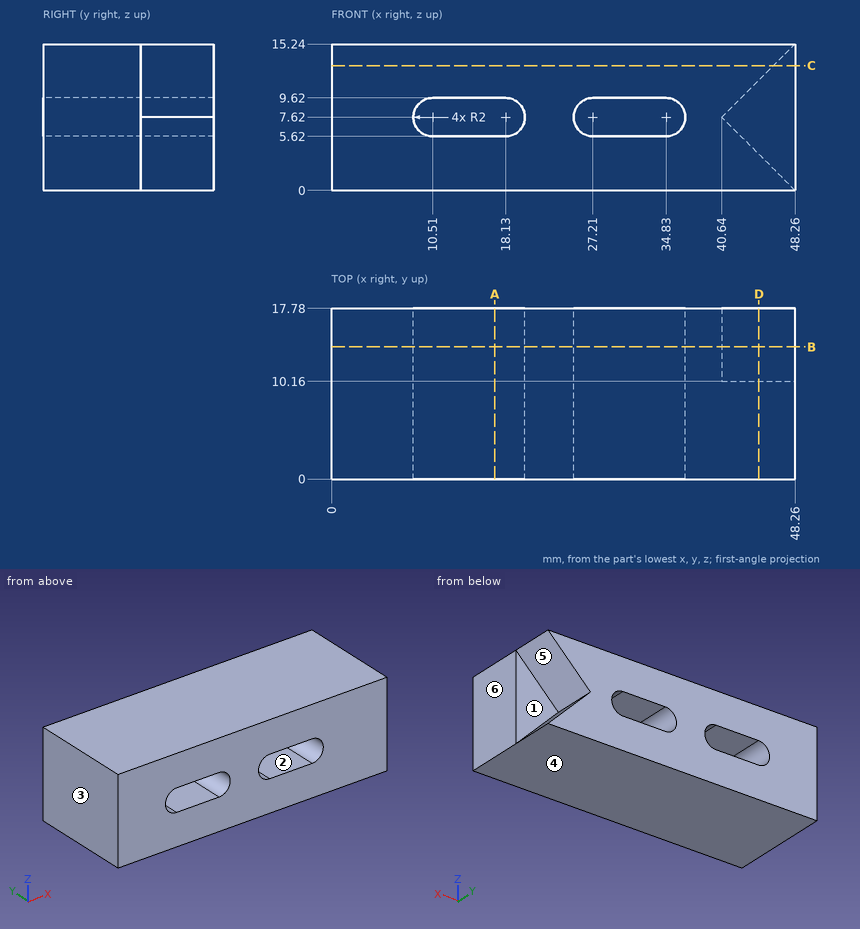
Part print with two shaded views. Sizes in mm from the minimum x, y, z corner. A direction names the side the tool comes from. Round coordinates to 2 decimals unless told otherwise and drop trailing zeros. Loops run counter-clockwise (first coordinate to the right, second up) from the corner with the lowest first, then second, coordinate; pieces in that order, holes last.
Item 1: Saw through at D-D (x = 44.5). List the corners of the cut face in (y, z).
Item 2: Drill centre lines: line 1 along Z through (x, y) = (33, 2.75); line 2 along X through (y, z) = (10.75, 6); line 3 along X through (y, z) = (7, 7.25). Where is each one in solid material? Low to high.
Item 3: Saw through at B-B (y = 13.75). List the corners of the cut face in (x, z), then the cut area to 3 significant figures.
Item 4: Saw through at C-C (z = 13). List the corners of the cut face in (x, y), then the cut area to 3 significant figures.
Item 5: Saw through at A-A (x = 17). List the corners of the cut face in (y, z).
Item 6: Two-plate mould, pull along Z, no slides. Class the marked faces 4, 5 and 6: released by +Z, released by -Z, zero draft, split by the parting line, or undercut.
Item 7: Which spindle directions (+Z, -Z, +X, -X, +Y, -Y) get a long thin tool onto all of the face, cutting with end or side? Do the marked faces 1, 2 and 3. Say none if no direction does.
Worked answers:
1. outline: (0, 0) - (17.78, 0) - (17.78, 3.76) - (10.16, 3.76) - (10.16, 11.48) - (17.78, 11.48) - (17.78, 15.24) - (0, 15.24) - close
2. line 1: z = 0 to 5.62, 9.62 to 15.24
2. line 2: x = 0 to 9.34, 19.3 to 26.04, 36 to 42.26
2. line 3: x = 0 to 8.54, 20.1 to 25.24, 36.8 to 48.26
3. outline: (0, 0) - (48.26, 0) - (40.64, 7.62) - (48.26, 15.24) - (0, 15.24) - close; hole (10.51, 5.62) - (18.13, 5.62) arc R2 ccw to (18.13, 9.62) - (10.51, 9.62) arc R2 ccw to start; hole (27.21, 5.62) - (34.83, 5.62) arc R2 ccw to (34.83, 9.62) - (27.21, 9.62) arc R2 ccw to start
3. area: 591 mm2
4. outline: (0, 0) - (48.26, 0) - (48.26, 10.16) - (46.02, 10.16) - (46.02, 17.78) - (0, 17.78) - close
4. area: 841 mm2
5. outline: (0, 0) - (17.78, 0) - (17.78, 5.62) - (0, 5.62) - close; (0, 9.62) - (17.78, 9.62) - (17.78, 15.24) - (0, 15.24) - close
6. face 4: released by -Z
6. face 5: undercut
6. face 6: zero draft
7. face 1: +X, +Y
7. face 2: +Y, -Y
7. face 3: +Z, -Z, -X, +Y, -Y
